```python
from build123d import *

# Parameters (mm, degrees)
F0_W       = 50.8
F0_H       = 50.8
F1_DEPTH   = 50.8
F2_W       = 49.4867833913
F2_H       = 49.351756752
F1_FACE1_W = 50.8
F1_FACE1_H = 50.8
F3_DEPTH   = 25.4
F4_DEPTH   = 69.85


with BuildPart() as f1:
    # F0 (on Front) → F1 (new body)
    with BuildSketch(Plane.XZ):
        with Locations((25.4, 25.4)):
            Rectangle(F0_W, F0_H)
    extrude(amount=F1_DEPTH)

    # F2 (on face) + F1_face1 (on face) → F3 (join)
    with BuildSketch(Plane(origin=(0, 0, 0), x_dir=(-1, 0, 0), z_dir=(0, 1, 0))):
        with Locations((-25.3845243424, 25.394623488)):
            Rectangle(F2_W, F2_H)
    with BuildSketch(Plane(origin=(25.4, -50.8, 25.4), x_dir=(1, 0, 0), z_dir=(0, -1, 0))):
        Rectangle(F1_FACE1_W, F1_FACE1_H)
    extrude(amount=F3_DEPTH, dir=(0, 1, 0))

    # F4 (cut): a face of the model
    f4_faces = [f1.faces().sort_by_distance(p)[0] for p in [
        (25.3845243424, 25.4, 25.394623488),
    ]]
    extrude(f4_faces, amount=-F4_DEPTH, mode=Mode.SUBTRACT)


solid = f1.part
```
CAD build for the part. Positions are in the model's coordinates, mm. A direction names the side the tool comes from. Coordinates: 2 decimals unless noted, no trailing zeros. Order: outer loops, then holes, each group sorted by start corner. A loop starts at its lowest first (then second) coordinate and runs counter-clockwise, first axis right, second up. Notation, with made-up numbers: (29.25, 33.5) - (47.25, 33.5) arc R12 cw to (47.25, 55.5) - close; hole circle Ø8 at (65, 47). An arc over 180 degrees is marked (long way). Answer in a Markdown table with one row per item.
1. Pull direction X, two halves, no side cores. Call faces 1 (the face through (0.641, -22, 25)), 2 (the face through (25, -25, 0)), 3 (the face through (50.8, -25, 25)), 4 (the face through (26, -22, 50.071)): +X half, -X half, draft (parallel to the pull), parting line (faces both ways), or undercut.
Answer:
| item | result |
|---|---|
| face 1 | undercut |
| face 2 | draft |
| face 3 | +X half |
| face 4 | undercut |
2. Slice it at B-B, the plane z = 32.5. List the corners of the cut face in (x, y).
Answer:
| item | result |
|---|---|
| outline | (0, -50.8) - (50.8, -50.8) - (50.8, 0) - (50.13, 0) - (50.13, -44.45) - (0.64, -44.45) - (0.64, 0) - (0, 0) - close |
3. 3-axis set-ups, long thin cutter, end or side, ignore diameter. For faces 5 (the face through (25, -25, 50.8)), 6 (the face through (26, -22, 0.719)): which of +Z, -Z, +X, -X, +Y, -Y reach the whole face in a straight line?
Answer:
| item | result |
|---|---|
| face 5 | +Z, +X, -X, +Y, -Y |
| face 6 | +Y |
4. Drill centre lines: L1, parallel to X at y = -43.5, z = 6; L2, parallel to Z at x = 36, y = -13; L3, parallel to Y at x = 37.5, z = 33. Where is each one in solid material? Low to high. Write a range as from..to.
Answer:
| item | result |
|---|---|
| L1 | 0..0.64, 50.13..50.8 |
| L2 | 0..0.72, 50.07..50.8 |
| L3 | -50.8..-44.45 |
5. Flat gauge pin, fed straight in: P1, Ø10, axis at x = 41.5, z = 27, coming from the +Y side. Where does the tip first touch, or does it go through?
Answer:
| item | result |
|---|---|
| P1 | y = -44.45 |
6. Slice it at C-C, the plane x = 4. List the corners of the cut face in (y, z), then the cut area to 3 significant figures.
Answer:
| item | result |
|---|---|
| outline | (-50.8, 0) - (0, 0) - (0, 0.72) - (-44.45, 0.72) - (-44.45, 50.07) - (0, 50.07) - (0, 50.8) - (-50.8, 50.8) - close |
| area | 387 mm² |
7. Slice it at A-A, the plane y = -23.5. List the corners of the cut face in (x, z), then the cut area to 3 significant figures.
Answer:
| item | result |
|---|---|
| outline | (0, 0) - (50.8, 0) - (50.8, 50.8) - (0, 50.8) - close; hole (0.64, 0.72) - (50.13, 0.72) - (50.13, 50.07) - (0.64, 50.07) - close |
| area | 138 mm² |
